Check sheet for the drawn part. Datum: minimum x, y, z corner. Units: mm. Give positions to 0.01 mm unless a question says otherwise; leave off trailing zeros. Write each loop counter-clockwise with the first axis right and the second up, starting at its lowest first coordinate (ties: lowest second). Pieces come first, ordered by that corner, then holes. Notation, with made-up numbers: (49, 75) - (92, 75) arc R15 ccw to (92, 103) - close; hole circle Ø2 at (-4, 47). An arc over 180 degrees is marked (long way). Use a Markdown table: item, result.
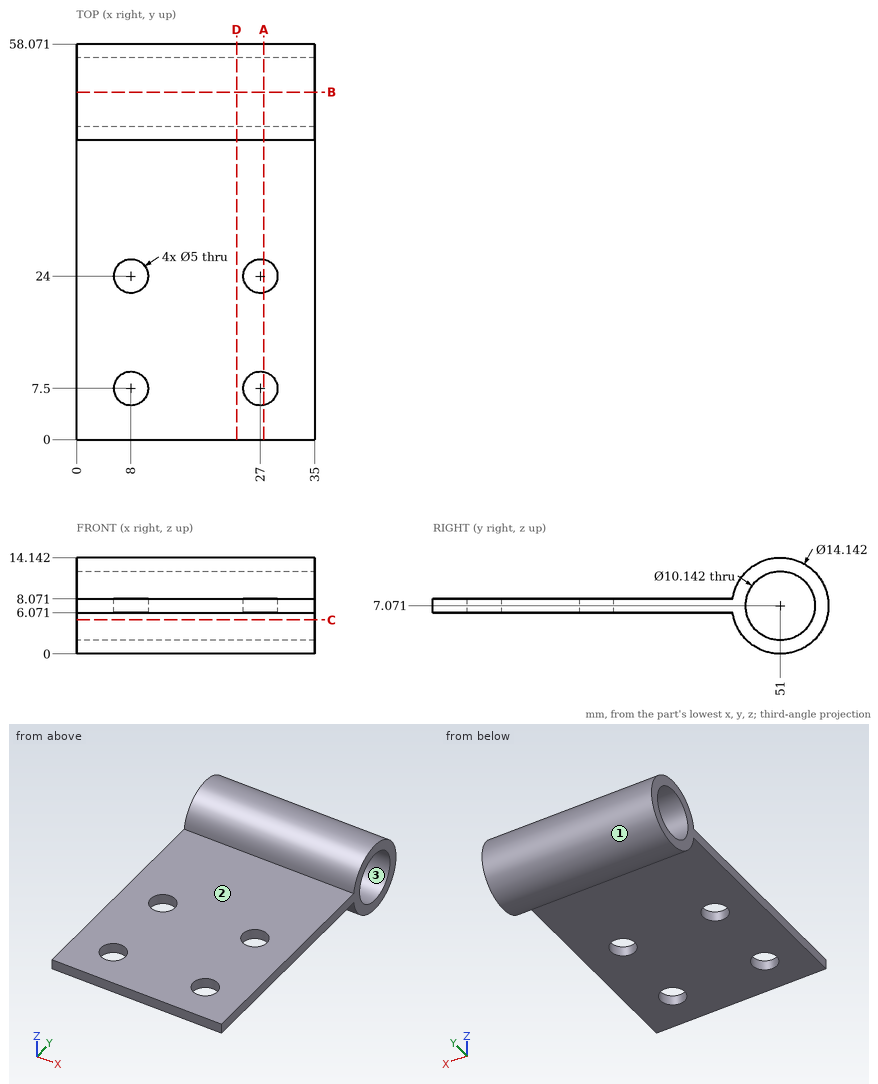
1) Section check B-B on y = 51. Record the boundary of the cut face in (x, z), then the cut area to 3 significant figures.
Working result:
| item | result |
|---|---|
| outline | (0, 0) - (35, 0) - (35, 2) - (0, 2) - close; (0, 12.14) - (35, 12.14) - (35, 14.14) - (0, 14.14) - close |
| area | 140 mm² |
2) Depth check by flat-ended pin: P1, Ø10, axis at x = 25.5, y = 36.5, coming from the -Z side; P2, Ø1, axis at x = 7.5, z = 11, coming from the -Y side; P3, Ø4, axis at x = 8, y = 7.5, coming from the -Z side; P4, Ø1.5, axis at x = 22, y = 35, coming from the +Z side. Enter the tip coordinate at first touch or a pass-through.
Working result:
| item | result |
|---|---|
| P1 | stops at z = 6.07 |
| P2 | stops at y = 44.82 |
| P3 | passes through |
| P4 | stops at z = 8.07 |
3) Section check D-D on x = 23.5. Record the boundary of the cut face in (y, z).
Working result:
| item | result |
|---|---|
| outline | (0, 6.07) - (44, 6.07) arc R7.07 ccw (long way) to (44, 8.07) - (0, 8.07) - close; hole circle Ø10.14 at (51, 7.07) |
4) Material ranges on L1, parallel to Y at x = 27, z = 7.4; L2, parallel to Y at x = 11, z = 6.75; L3, parallel to Y at x = 3.5, z = 4.75, recorded low to high. Write a range as from..to.
Working result:
| item | result |
|---|---|
| L1 | y = 0..5, 10..21.5, 26.5..45.94, 56.06..58.06 |
| L2 | y = 0..45.94, 56.06..58.06 |
| L3 | y = 44.32..46.49, 55.51..57.68 |
5) Section check C-C on z = 5. Record the boundary of the cut face in (x, y).
Working result:
| item | result |
|---|---|
| outline | (0, 44.24) - (35, 44.24) - (35, 46.37) - (0, 46.37) - close; (0, 55.63) - (35, 55.63) - (35, 57.76) - (0, 57.76) - close |
6) Mould release check, pull along Y, two halves, no side actions. Record for the marked faces 1, 2 and 3: pulls with the +Y half, pulls with the -Y half, needs draft (parallel to the pull), parting line crosses it, or undercut.
Working result:
| item | result |
|---|---|
| face 1 | parting line crosses it |
| face 2 | needs draft |
| face 3 | undercut |
7) Section check A-A on x = 27.5. Record the boundary of the cut face in (y, z).
Working result:
| item | result |
|---|---|
| outline | (0, 6.07) - (5.05, 6.07) - (5.05, 8.07) - (0, 8.07) - close; (9.95, 6.07) - (21.55, 6.07) - (21.55, 8.07) - (9.95, 8.07) - close; (26.45, 6.07) - (44, 6.07) arc R7.07 ccw (long way) to (44, 8.07) - (26.45, 8.07) - close; hole circle Ø10.14 at (51, 7.07) |
